```python
from build123d import *

# Parameters (mm, degrees)
F0_R     = 6
F1_DEPTH = 18
F3_D     = 4.3


with BuildPart() as f1:
    # F0 (on Front) → F1 (new body, symmetric)
    with BuildSketch(Plane.XZ):
        Polygon((21, 15), (-21, 15), (-21, -9), (-10, -9), (-5, -13), (0, -13), (5, -13), (10, -9), (21, -9), align=None)
        Circle(F0_R, mode=Mode.SUBTRACT)
    extrude(amount=F1_DEPTH, both=True)

    # F3 (through all)
    with Locations(Plane.XY.offset(15)):
        with Locations((-15.25, 13), (15.25, 13), (15.25, -13), (-15.25, -13)):
            Hole(F3_D / 2)


solid = f1.part
```
The model under review builds one solid part; all positions refer to its coordinate system, in mm. A direction names the side the tool comes from. Round coordinates to 2 decimals unless told otherwise and drop trailing zeros. Order: outer loops, then holes, each group sorted by start corner. A loop starts at its lowest first (then second) coordinate and runs counter-clockwise, first axis right, second up.
Item 1: Add section C-C, the plane y = -3.5. State the section outline as (x, z) points, and give its area (3 significant figures).
Working result:
outline: (-21, -9) - (-10, -9) - (-5, -13) - (5, -13) - (10, -9) - (21, -9) - (21, 15) - (-21, 15) - close; hole circle Ø12 at (0, 0)
area: 955 mm2
Item 2: To check wall thickness, follow probe 1 along Y at (x, z) = (15.25, 3.5); probe 2 along Y at (x, z) = (13.5, -2.5); probe 3 along Z at (x, y) = (0, 9). State the ranges of each line that lie inside material, in increasing order.
Working result:
probe 1: y = -18 to -15.15, -10.85 to 10.85, 15.15 to 18
probe 2: y = -18 to -14.25, -11.75 to 11.75, 14.25 to 18
probe 3: z = -13 to -6, 6 to 15
Item 3: Draft analysis for pull direction Z (two halves, no side actions). For faces 3 (the flat face through (0, 0, 15)), 4 (the cylindrical face through (-6, 0, 0)), 5 (the flat face through (21, 0, 3)), 6 (the flat face through (-16, 0, -9)), state which applies: released by +Z, released by -Z, zero draft, split by the parting line, or undercut.
Working result:
face 3: released by +Z
face 4: undercut
face 5: zero draft
face 6: released by -Z
Item 4: Add section D-D, the plane x = 15.25. State the section outline as (y, z) points, and give its area (3 significant figures).
Working result:
outline: (-18, -9) - (-15.15, -9) - (-15.15, 15) - (-18, 15) - close; (-10.85, -9) - (10.85, -9) - (10.85, 15) - (-10.85, 15) - close; (15.15, -9) - (18, -9) - (18, 15) - (15.15, 15) - close
area: 658 mm2
Item 5: Add section B-B, the plane z = 5.5. State the section outline as (x, y) points, and give its area (3 significant figures).
Working result:
outline: (-21, -18) - (-2.4, -18) - (-2.4, 18) - (-21, 18) - close; (2.4, -18) - (21, -18) - (21, 18) - (2.4, 18) - close; hole circle Ø4.3 at (-15.25, -13); hole circle Ø4.3 at (-15.25, 13); hole circle Ø4.3 at (15.25, -13); hole circle Ø4.3 at (15.25, 13)
area: 1,280 mm2
Item 6: Machinability: for faces 1 (the flat face through (0, -18, 7)), 2 (the flat face through (15, 0, -9)), which of the approach directions +Z, -Z, +X, -X, +Y, -Y give a long, thin tool a straight path to every point of the face, cutting with its end or side? Answer none if there is none.
Working result:
face 1: +Z, -Z, +X, -X, -Y
face 2: -Z, +X, +Y, -Y
Item 7: For pin 1 (5.5 mm diameter, centred on x = -15.25, y = -13, fed in from +Z); pin 2 (5 mm diameter, centred on x = 8.5, y = 2.5, fed in from -Z); pin 3 (9 mm diameter, centred on x = 18, y = -9, fed in from -Z), all flat-tipped, find the tip position at first contact; note any pin that passes through.
Working result:
pin 1: stops at z = 15
pin 2: stops at z = -12.2
pin 3: stops at z = -9
Item 8: Add section A-A, the plane y = 13. State the section outline as (x, z) points.
Working result:
outline: (-21, -9) - (-17.4, -9) - (-17.4, 15) - (-21, 15) - close; (-13.1, -9) - (-10, -9) - (-5, -13) - (5, -13) - (10, -9) - (13.1, -9) - (13.1, 15) - (-13.1, 15) - close; (17.4, -9) - (21, -9) - (21, 15) - (17.4, 15) - close; hole circle Ø12 at (0, 0)
